The listing builds one solid part. Answer for the finished solid, in the listing's coordinates (mm). Round coordinates to 2 decimals unless told otherwise and drop trailing zeros. Loops run counter-clockwise (first coordinate to the right, second up) from the corner with the lowest first, then second, coordinate; pieces in that order, holes last. Notation, with made-up numbers: (88.5, 88.25) -> (131.5, 88.25) arc R23 ccw to (131.5, 123.25) -> close; hole circle Ø2 at (-37.5, 45). An arc over 180 degrees is marked (long way). One line per question, with ' | ' between items.
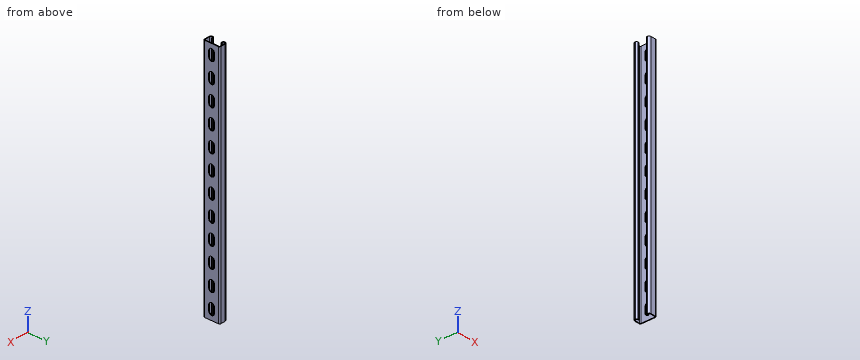
from build123d import *

# Parameters (mm, degrees)
BOSS_EXTRUDE1_DEPTH = 609.6
CUT_EXTRUDE1_DEPTH  = 1.778
LPATTERN1_COUNT     = 12
LPATTERN1_PITCH     = 50.8


with BuildPart() as part:
    # Sketch1 → Boss-Extrude1 (new body)
    with BuildSketch(Plane.XY):
        with BuildLine():
            Line((-15.58925, 20.6375), (-3.46075, 20.6375))
            ThreePointArc((-3.46075, 20.6375), (-1.013630207, 19.623869793), (0, 17.17675))
            Line((0, 17.17675), (0, -17.17675))
            ThreePointArc((0, -17.17675), (-1.013630207, -19.623869793), (-3.46075, -20.6375))
            Line((-3.46075, -20.6375), (-15.58925, -20.6375))
            ThreePointArc((-15.58925, -20.6375), (-19.158901808, -19.158901808), (-20.6375, -15.58925))
            Line((-20.6375, -15.58925), (-20.6375, -14.57325))
            ThreePointArc((-20.6375, -14.57325), (-19.623869793, -12.126130207), (-17.17675, -11.1125))
            Line((-17.17675, -11.1125), (-14.3891, -11.1125))
            ThreePointArc((-14.3891, -11.1125), (-13.5001, -12.0015), (-14.3891, -12.8905))
            Line((-14.3891, -12.8905), (-17.17675, -12.8905))
            ThreePointArc((-17.17675, -12.8905), (-18.366633936, -13.383366064), (-18.8595, -14.57325))
            Line((-18.8595, -14.57325), (-18.8595, -15.58925))
            ThreePointArc((-18.8595, -15.58925), (-17.901665951, -17.901665951), (-15.58925, -18.8595))
            Line((-15.58925, -18.8595), (-3.46075, -18.8595))
            ThreePointArc((-3.46075, -18.8595), (-2.270866064, -18.366633936), (-1.778, -17.17675))
            Line((-1.778, -17.17675), (-1.778, 17.17675))
            ThreePointArc((-1.778, 17.17675), (-2.270866064, 18.366633936), (-3.46075, 18.8595))
            Line((-3.46075, 18.8595), (-15.58925, 18.8595))
            ThreePointArc((-15.58925, 18.8595), (-17.901665951, 17.901665951), (-18.8595, 15.58925))
            Line((-18.8595, 15.58925), (-18.8595, 14.57325))
            ThreePointArc((-18.8595, 14.57325), (-18.366633936, 13.383366064), (-17.17675, 12.8905))
            Line((-17.17675, 12.8905), (-14.3891, 12.8905))
            ThreePointArc((-14.3891, 12.8905), (-13.5001, 12.0015), (-14.3891, 11.1125))
            Line((-14.3891, 11.1125), (-17.17675, 11.1125))
            ThreePointArc((-17.17675, 11.1125), (-19.623869793, 12.126130207), (-20.6375, 14.57325))
            Line((-20.6375, 14.57325), (-20.6375, 15.58925))
            ThreePointArc((-20.6375, 15.58925), (-19.158901808, 19.158901808), (-15.58925, 20.6375))
        make_face()
    extrude(amount=-BOSS_EXTRUDE1_DEPTH)

    # Sketch2 → Cut-Extrude1 (cut)
    with BuildSketch(Plane(origin=(0, 0, 0), x_dir=(0, 0, -1), z_dir=(1, 0, 0))):
        with BuildLine():
            Line((18.25625, 7.14375), (32.54375, 7.14375))
            ThreePointArc((32.54375, 7.14375), (39.6875, 0), (32.54375, -7.14375))
            Line((32.54375, -7.14375), (18.25625, -7.14375))
            ThreePointArc((18.25625, -7.14375), (11.1125, 0), (18.25625, 7.14375))
        make_face()
    cut_extrude1 = extrude(amount=-CUT_EXTRUDE1_DEPTH, mode=Mode.SUBTRACT)

    # LPattern1: Cut-Extrude1 ×12
    with Locations(*[(0, 0, -i * LPATTERN1_PITCH) for i in range(1, LPATTERN1_COUNT)]):
        add(cut_extrude1, mode=Mode.SUBTRACT)


solid = part.part
Q1. A cutting plane is placed at D-D on y = 0. Give the number of separate pieces and of enclosed holes in the cut face, plus the area to 3 significant figures.
Numbers:
separate pieces: 13 | enclosed holes: 0 | area: 474 mm^2
Q2. A cutting plane is placed at C-C on z = -355.5. Give the vertices of the cut face in (x, y), plus the area to 3 significant figures.
Numbers:
outline: (-20.64, -15.59) arc R5.05 ccw to (-15.59, -20.64) -> (-3.46, -20.64) arc R3.46 ccw to (0, -17.18) -> (0, 17.18) arc R3.46 ccw to (-3.46, 20.64) -> (-15.59, 20.64) arc R5.05 ccw to (-20.64, 15.59) -> (-20.64, 14.57) arc R3.46 ccw to (-17.18, 11.11) -> (-14.39, 11.11) arc R0.89 ccw to (-14.39, 12.89) -> (-17.18, 12.89) arc R1.68 cw to (-18.86, 14.57) -> (-18.86, 15.59) arc R3.27 cw to (-15.59, 18.86) -> (-3.46, 18.86) arc R1.68 cw to (-1.78, 17.18) -> (-1.78, -17.18) arc R1.68 cw to (-3.46, -18.86) -> (-15.59, -18.86) arc R3.27 cw to (-18.86, -15.59) -> (-18.86, -14.57) arc R1.68 cw to (-17.18, -12.89) -> (-14.39, -12.89) arc R0.89 ccw to (-14.39, -11.11) -> (-17.18, -11.11) arc R3.46 ccw to (-20.64, -14.57) -> close | area: 172 mm^2
Q3. A cutting plane is placed at A-A on x = -7.75. Give the vertices of the cut face in (y, z).
Numbers:
outline: (-20.64, -609.6) -> (-18.86, -609.6) -> (-18.86, 0) -> (-20.64, 0) -> close; (18.86, -609.6) -> (20.64, -609.6) -> (20.64, 0) -> (18.86, 0) -> close
Q4. Given pin 1 Ø0.9 at (x, z) = (-1, -333) entering from +Y; pin 2 Ø2 at (x, z) = (-1.5, -587) entering from -Y; pin 3 Ø1.4 at (x, z) = (-0.5, -379) entering from -Y, each flat-ended and moving along its own axis, determine where each tip first touches the part or whether it passes through.
Numbers:
pin 1: y = 19.99 | pin 2: y = -20.5 | pin 3: y = -19.8
Q5. Find the intervals of material crossed by line 1 (Y direction, x = -15.5, z = -106.5); line 2 (Y direction, x = -13, z = -407); line 3 (X direction, y = 16, z = -385.5), in increasing order. Write a range as from..to.
Numbers:
line 1: -20.64..-18.86, -12.89..-11.11, 11.11..12.89, 18.86..20.64 | line 2: -20.64..-18.86, 18.86..20.64 | line 3: -20.62..-18.83, -1.78..0
